Read the model definition and answer for the solid it produces. Units are mm, in the model's axes. Coordinates: 2 decimals unless noted, no trailing zeros. Order: outer loops, then holes, each group sorted by start corner. A loop starts at its lowest first (then second) coordinate and runs counter-clockwise, first axis right, second up.
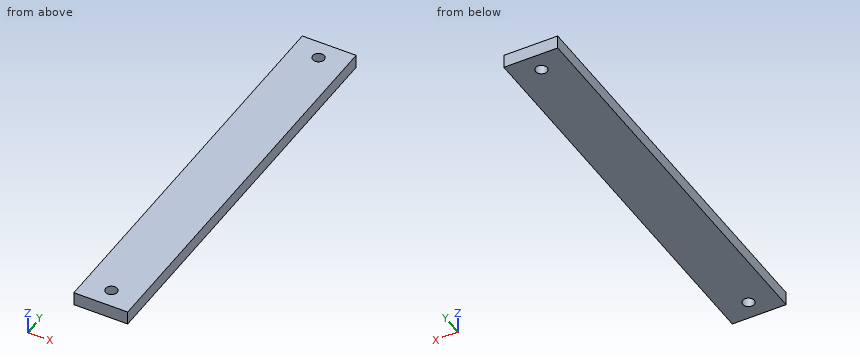
Autodesk Inventor part; units mm, degrees
ref_plane "YZ Plane" through (0, 0, 0) normal (1, 0, 0) x (0, 1, 0)
ref_plane "XZ Plane" through (0, 0, 0) normal (0, 1, 0) x (-1, 0, 0)
ref_plane "XY Plane" through (0, 0, 0) normal (0, 0, 1) x (1, 0, 0)
sketch "Náčrt1" plane through (0, 0, 0) normal (0, 0, 1) x (1, 0, 0)
  line L0 (0, 52.5) -> (0, -52.5)
  line L1 (-7, 0) -> (7, 0)
  line L2 (-5, 37.5) -> (5, 37.5)
  line L3 (5, 37.5) -> (5, -37.5)
  line L4 (5, -37.5) -> (-5, -37.5)
  line L5 (-5, -37.5) -> (-5, 37.5)
  point P0 (0, 0)
  dimension "d0" = 75
  dimension "d1" = 10
extrude "Vysunutí1" add sketch "Náčrt1" along normal blind 2.5
sketch "Náčrt2" plane through (0, 0, 2.5) normal (0, 0, 1) x (1, 0, 0)
  line L0 (0, 52.5) -> (0, -52.5)
  line L1 (-7, 0) -> (7, 0)
  line L2 (-5, -37.5) -> (5, -37.5)
  line L3 (5, -37.5) -> (5, 37.5)
  line L4 (5, 37.5) -> (-5, 37.5)
  line L5 (-5, 37.5) -> (-5, -37.5)
  point P0 (0, 0)
  point P1 (0, 34)
  point P2 (0, -34)
  dimension "d4" = 3.5
  dimension "d5" = 3.5
hole "Díra1" at (0, 34, 2.5) at (0, -34, 2.5) direction (0, 0, -1) diameter 2.15 end through all
properties part number "battery_plate_3D tisk"
1) A cutting plane is placed at B-B, the plane x = 0. Determine the outline of the cut face in (y, z) (3 decimals), and give its area (3 significant figures).
A:
outline: (-37.5, 0) - (-35.075, 0) - (-35.075, 2.5) - (-37.5, 2.5) - close; (-32.925, 0) - (32.925, 0) - (32.925, 2.5) - (-32.925, 2.5) - close; (35.075, 0) - (37.5, 0) - (37.5, 2.5) - (35.075, 2.5) - close
area: 177 mm2
2) Straight lines are drawn through the part: line 1 (Y direction, x = 0, z = 1.8) (3 decimals); line 2 (X direction, y = -34, z = 0.5) (3 decimals); line 3 (Y direction, x = 0.25, z = 0.2). For each, find the intervals that lie inside material, in ascending order.
A:
line 1: y = -37.5 to -35.075, -32.925 to 32.925, 35.075 to 37.5
line 2: x = -5 to -1.075, 1.075 to 5
line 3: y = -37.5 to -35.05, -32.95 to 32.95, 35.05 to 37.5
3) A cutting plane is placed at A-A, the plane y = -34. Determine the outline of the cut face in (x, z) (3 decimals).
A:
outline: (-5, 0) - (-1.075, 0) - (-1.075, 2.5) - (-5, 2.5) - close; (1.075, 0) - (5, 0) - (5, 2.5) - (1.075, 2.5) - close
